Could you check a few things on this model? Use its own coordinates, in mm. Give positions to 0.01 mm unless a question says otherwise; leave off trailing zeros. Loops run counter-clockwise (first coordinate to the right, second up) from the corner with the lowest first, then second, coordinate; pieces in that order, holes last. Notation, with made-up numbers: (-3.75, 74) - (8.25, 74) arc R30 cw to (8.25, 106) - close; hole circle Ø11 at (39.5, 81.25). An arc over 180 degrees is marked (long way). Write each question's results on one line, items separated by ' | '. Start each with the question number.
1) I want a section at D-D, the plane x = -45. Write out the boundary of the cut face in (y, z), and give its area (4 significant figures).
2) If I drill on probe 1 along X at (y, z) = (-0.25, 1.95); probe 2 along Y at (x, z) = (35.5, 0.8); probe 3 along Y at (x, z) = (-45, 2.5), over which ranges is the centre line in solid material (lowest first)? Write a range as [from, to].
3) I want a section at C-C, the plane z = 3.7. Write out the boundary of the cut face in (x, y), and give its area (3 significant figures).
4) I want a section at B-B, the plane y = 0. Write out the boundary of the cut face in (x, z), and give its area (3 significant figures).
5) I'm going to push a flat-ended pin straight in: pin 1 (1.7 mm diameter, centred on x = -34, y = 1, fed in from +Z). Where does the tip first touch, or does it pass through?
6) I want a section at A-A, the plane x = -10. Write out the boundary of the cut face in (y, z).
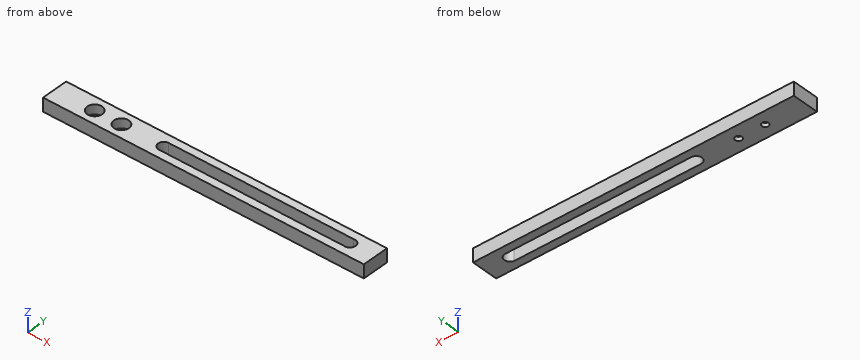
from build123d import *

# Parameters (mm, degrees)
SKETCH_1_W          = 120
SKETCH_1_H          = 10
EXTRUDE_1_DEPTH     = 5
SKETCH_2_R          = 1.25
CUT_EXTRUDE_1_DEPTH = 5
SKETCH_3_R          = 2.8
CUT_EXTRUDE_2_DEPTH = 3.5


with BuildPart() as part:
    # Эскиз1 → Бобышка-Вытянуть1 (new body)
    with BuildSketch(Plane.XY):
        Rectangle(SKETCH_1_W, SKETCH_1_H)
    extrude(amount=EXTRUDE_1_DEPTH)

    # Эскиз2 → Вырез-Вытянуть1 (cut)
    with BuildSketch(Plane.XY.offset(5)):
        with Locations((-45, 0)):
            Circle(SKETCH_2_R)
        with Locations((-35, 0)):
            Circle(SKETCH_2_R)
        with BuildLine():
            Line((-19.160353307, 2.1), (50, 2.1))
            ThreePointArc((50, 2.1), (52.519823346, 0.419823346), (50.839646693, -2.1))
            Line((50.839646693, -2.1), (-19.160353307, -2.1))
            ThreePointArc((-19.160353307, -2.1), (-21.260353307, 0), (-19.160353307, 2.1))
        make_face()
    extrude(amount=-CUT_EXTRUDE_1_DEPTH, mode=Mode.SUBTRACT)

    # Эскиз3 → Вырез-Вытянуть2 (cut)
    with BuildSketch(Plane.XY.offset(5)):
        with Locations((-45, 0)):
            Circle(SKETCH_3_R)
        with Locations((-35, 0)):
            Circle(SKETCH_3_R)
    extrude(amount=-CUT_EXTRUDE_2_DEPTH, mode=Mode.SUBTRACT)


solid = part.part
Answers:
1) outline: (-5, 0) - (-1.25, 0) - (-1.25, 1.5) - (-2.8, 1.5) - (-2.8, 5) - (-5, 5) - close; (1.25, 0) - (5, 0) - (5, 5) - (2.8, 5) - (2.8, 1.5) - (1.25, 1.5) - close | area: 26.65 mm2
2) probe 1: x = [-60, -47.79], [-42.21, -37.79], [-32.21, -21.25], [52.55, 60] | probe 2: y = [-5, -2.1], [2.1, 5] | probe 3: y = [-5, -2.8], [2.8, 5]
3) outline: (-60, -5) - (60, -5) - (60, 5) - (-60, 5) - close; hole circle Ø5.6 at (-45, 0); hole circle Ø5.6 at (-35, 0); hole (-19.16, -2.1) - (50.84, -2.1) arc R2.14 ccw to (50, 2.1) - (-19.16, 2.1) arc R2.1 ccw to start | area: 844 mm2
4) outline: (-60, 0) - (-46.25, 0) - (-46.25, 1.5) - (-47.8, 1.5) - (-47.8, 5) - (-60, 5) - close; (-43.75, 0) - (-36.25, 0) - (-36.25, 1.5) - (-37.8, 1.5) - (-37.8, 5) - (-42.2, 5) - (-42.2, 1.5) - (-43.75, 1.5) - close; (-33.75, 0) - (-21.26, 0) - (-21.26, 5) - (-32.2, 5) - (-32.2, 1.5) - (-33.75, 1.5) - close; (52.56, 0) - (60, 0) - (60, 5) - (52.56, 5) - close | area: 184 mm2
5) pin 1: stops at z = 1.5
6) outline: (-5, 0) - (-2.1, 0) - (-2.1, 5) - (-5, 5) - close; (2.1, 0) - (5, 0) - (5, 5) - (2.1, 5) - close
